Model file for the job. Use its own axes, mm. A direction names the side the tool comes from. Round coordinates to 2 decimals unless told otherwise and drop trailing zeros. Order: outer loops, then holes, each group sorted by start corner. A loop starts at its lowest first (then second) coordinate and runs counter-clockwise, first axis right, second up. Notation, with made-up numbers: (-34.5, -11.5) -> (-5.5, -11.5) arc R7 ccw to (-5.5, -1.5) -> close; hole circle Ø7 at (0.25, 28.5). An arc over 180 degrees is marked (long way). Put each result on its own line as item: value. Start each with the question number.
Q1. Flat gauge pins, fed straight in: P1, Ø1.8, axis at y = 1.5, z = 2, coming from the +X side; P2, Ø0.7, axis at y = 14, z = 2, coming from the +X side; P3, Ø1.5, axis at x = -1.5, y = 5.5, coming from the -Z side; P4, Ø1.1, axis at y = 1.5, z = 2, coming from the -X side. Where does each tip first touch, or does it go through?
Q2. Probe L1, parallel to Y at x = 0, z = 0.5; L2, parallel to Y at x = 10, z = 2; L3, parallel to X at y = 13, z = 1.9. List the from-to ranges inside material, lowest first.
Q3. Cut at D-D, the plane z = 0.8. List the corners of the cut face in (x, y), and give its area (3 significant figures).
Q4. 3-axis set-ups, long thin cutter, end or side, ignore diameter. For faces 1 (the face through (3, 11, 0)), 2 (the face through (3.5, 1, 2)), 3 (the face through (0, 12, 1.3)), 4 (the face through (-8, 3.549, 2)): which of +Z, -Z, +X, -X, +Y, -Y reach the whole face in a straight line?
Q5. Pull direction X, two halves, no side cores. Call faces 5 (the face through (5, 13, 3.5)), 6 (the face through (3.5, 14, 2)), 7 (the face through (-13.25, -0.42, 1.73)): released by +X, released by -X, zero draft, split by the parting line, or undercut.
Q6. Cut at B-B, the plane z = 3.05. List the corners of the cut face in (x, y) (3 decimals), and give its area (3 significant figures).
Q7. Cut at C-C, the plane y = 2. List the corners of the cut face in (x, z), and give its area (3 significant figures).
Q8. Cut at A-A, the plane x = 0. List the corners of the cut face in (y, z).
from build123d import *

# Parameters (mm, degrees)
EXTRUDE_1_DEPTH     = 3.5
EXTRUDE_8_DEPTH     = 3.5
SKETCH_12_R         = 4
CUT_EXTRUDE_1_DEPTH = 27.432726041
SKETCH_13_R         = 5.325
CUT_EXTRUDE_2_DEPTH = 2.2
CUT_EXTRUDE_3_DEPTH = 2.2


with BuildPart() as part:
    # ｽｹｯﾁ1 → ﾎﾞｽ - 押し出し1 (new body)
    with BuildSketch(Plane.XY):
        Polygon((0, 21.650635095), (-12.5, 0), (12.5, 0), align=None)
    extrude(amount=EXTRUDE_1_DEPTH)

    # ｽｹｯﾁ11 → ﾎﾞｽ - 押し出し8 (add, through all)
    with BuildSketch(Plane(origin=(0, 0, 0), x_dir=(-1, 0, 0), z_dir=(0, 0, -1))):
        with BuildLine():
            Line((0.866025404, 22.150635095), (13.366025404, 0.5))
            ThreePointArc((13.366025404, 0.5), (13.243672874, -0.429359734), (12.5, -1))
            Line((12.5, -1), (-12.5, -1))
            ThreePointArc((-12.5, -1), (-13.243672874, -0.429359734), (-13.366025404, 0.5))
            Line((-13.366025404, 0.5), (-0.866025404, 22.150635095))
            ThreePointArc((-0.866025404, 22.150635095), (0, 22.509354562), (0.866025404, 22.150635095))
        make_face()
        Polygon((0, 21.650635095), (12.5, 0), (-12.5, 0), align=None, mode=Mode.SUBTRACT)
    extrude(amount=-EXTRUDE_8_DEPTH)

    # ｽｹｯﾁ12 → ｶｯﾄ - 押し出し1 (cut, through all)
    with BuildSketch(Plane.XY.offset(3.5)):
        with Locations((0, 7.24327674)):
            Circle(SKETCH_12_R)
    extrude(amount=-CUT_EXTRUDE_1_DEPTH, mode=Mode.SUBTRACT)

    # ｽｹｯﾁ13 → ｶｯﾄ - 押し出し2 (cut)
    with BuildSketch(Plane.XY.offset(3.5)):
        with Locations((0, 7.048781332)):
            Circle(SKETCH_13_R)
    extrude(amount=-CUT_EXTRUDE_2_DEPTH, mode=Mode.SUBTRACT)

    # ｽｹｯﾁ14 → ｶｯﾄ - 押し出し3 (cut)
    with BuildSketch(Plane.XY.offset(3.5)):
        Polygon((-3.5, 24.86994882), (3.5, 24.86994882), (3.5, 10.548781332), (20.875633237, 10.548781332), (20.875633237, 3.548781332), (3.5, 3.548781332), (3.5, -2.871018352), (-3.5, -2.871018352), (-3.5, 3.548781332), (-19.259035821, 3.548781332), (-19.259035821, 10.548781332), (-3.5, 10.548781332), align=None)
    extrude(amount=-CUT_EXTRUDE_3_DEPTH, mode=Mode.SUBTRACT)


solid = part.part
Ans:
1. P1: stops at x = 13.31
1. P2: stops at x = 5.77
1. P3: passes through
1. P4: stops at x = -13.11
2. L1: y = -1 to 3.24, 11.24 to 22.51
2. L2: y = -1 to 3.55
2. L3: x = -6.15 to -3.5, 3.5 to 6.15
3. outline: (-13.37, 0.5) arc R1.22 ccw to (-12.5, -1) -> (12.5, -1) arc R1.22 ccw to (13.37, 0.5) -> (0.87, 22.15) arc R1.22 ccw to (-0.87, 22.15) -> close; hole circle Ø8 at (0, 7.24)
3. area: 298 mm^2
4. face 1: -Z, +X, -X, +Y, -Y
4. face 2: +Z, +Y, -Y
4. face 3: +Z
4. face 4: +Z, +X, -X
5. face 5: zero draft
5. face 6: undercut
5. face 7: released by -X
6. outline: (-13.366, 0.5) arc R1.225 ccw to (-12.5, -1) -> (-3.5, -1) -> (-3.5, 3.036) arc R5.325 cw to (-4.013, 3.549) -> (-11.606, 3.549) -> close; (-7.564, 10.549) -> (-4.013, 10.549) arc R5.325 cw to (-3.5, 11.062) -> (-3.5, 17.588) -> close; (3.5, -1) -> (12.5, -1) arc R1.225 ccw to (13.366, 0.5) -> (11.606, 3.549) -> (4.013, 3.549) arc R5.325 cw to (3.5, 3.036) -> close; (3.5, 11.062) arc R5.325 cw to (4.013, 10.549) -> (7.564, 10.549) -> (3.5, 17.588) -> close
6. area: 112 mm^2
7. outline: (-12.5, 0) -> (12.5, 0) -> (12.5, 3.5) -> (3.5, 3.5) -> (3.5, 1.3) -> (-3.5, 1.3) -> (-3.5, 3.5) -> (-12.5, 3.5) -> close
7. area: 72.1 mm^2
8. outline: (-1, 0) -> (3.24, 0) -> (3.24, 1.3) -> (-1, 1.3) -> close; (11.24, 0) -> (22.51, 0) -> (22.51, 1.3) -> (11.24, 1.3) -> close
